Verification items for the finished model (mm, model axes). Face numbers are marked on the shaded views. Give positions to 0.01 mm unless a question says otherwise; leave off trailing zeros. Order: outer loops, then holes, each group sorted by start corner. A loop starts at its lowest first (then second) coordinate and runs counter-clockwise, first axis right, second up. Notation, with made-up numbers: (17.5, -37) -> (41.5, -37) arc R25 cw to (41.5, -16) -> close; hole circle Ø6 at (65, -8). An arc over 180 degrees is marked (long way). One line per question, with ' | ' between items. Start each with the question number.
Q1. Section check D-D on y = 12.75. Record the cut outline in (x, z), plus the area to 3 significant figures.
Q2. Section check C-C on z = 0. Record the cut outline in (x, y), plus the area to 3 significant figures.
Q3. Section check B-B on z = -20. Record the cut outline in (x, y), plus the area to 3 significant figures.
Q4. Material ranges on probe 1 along Z at (x, y) = (-2, 20.5); probe 2 along Y at (x, z) = (3.25, 0); probe 3 along Y at (x, z) = (4.75, -4), recorded low to high. Write a range as [from, to].
Q5. Go/stop test with flat-tipped pins: pin 1 (1 mm diameter, centred on x = 1.5, y = 17.5, fed in from +Z); pin 2 (1.3 mm diameter, centred on y = 20, z = -31, fed in from -X); pin 3 (8 mm diameter, centred on y = 6, z = -43, fed in from -X). Record where each tip stops, or that it passes through.
Q6. Section check A-A on z = 42. Record the cut outline in (x, y).
Q7. Mould release check, pull along X, two halves, no side actions. Record for the marked faces 1 and 2: released by +X, released by -X, zero draft, split by the parting line, or undercut.
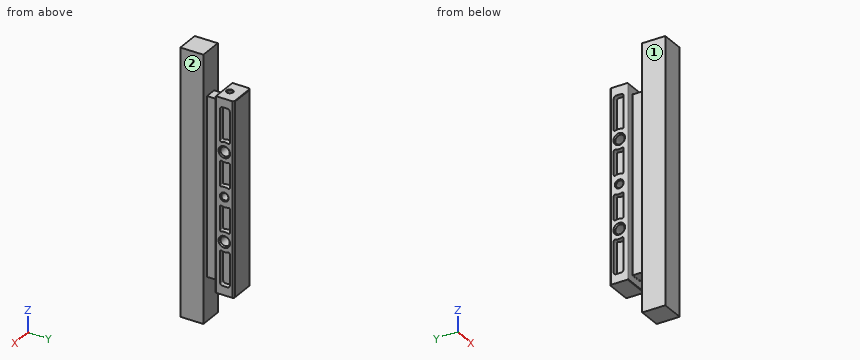
from build123d import *

# Parameters (mm, degrees)
BOSS_EXTRUDE1_DEPTH      = 60
BOSS_EXTRUDE1_DEPTH_BACK = 60
CUT_EXTRUDE1_DEPTH       = 12
CUT_EXTRUDE1_DEPTH_BACK  = 12
CUT_EXTRUDE2_DEPTH       = 2.3
CUT_EXTRUDE3_DEPTH       = 2.3
CUT_EXTRUDE4_DEPTH       = 2.3
CUT_EXTRUDE5_DEPTH       = 2.3
CUT_EXTRUDE6_DEPTH       = 2.3
CUT_EXTRUDE7_DEPTH       = 2.3
CUT_EXTRUDE8_DEPTH       = 2.3
CUT_EXTRUDE9_DEPTH       = 2.3


with BuildPart() as part:
    # Sketch1 → Boss-Extrude1 (new body, two sides)
    with BuildSketch(Plane.XY) as boss_extrude1_sk:
        with BuildLine():
            Line((-5.8, 16.5), (-2.9, 16.5))
            ThreePointArc((-2.9, 16.5), (-2.687867966, 16.412132034), (-2.6, 16.2))
            Line((-2.6, 16.2), (-2.6, 10.5))
            Line((-2.6, 10.5), (-5.25, 10.5))
            Line((-5.25, 10.5), (-5.25, 0))
            Line((-5.25, 0), (5.25, 0))
            Line((5.25, 0), (5.25, 10.5))
            Line((5.25, 10.5), (2.6, 10.5))
            Line((2.6, 10.5), (2.6, 16.2))
            ThreePointArc((2.6, 16.2), (2.687867966, 16.412132034), (2.9, 16.5))
            Line((2.9, 16.5), (5.8, 16.5))
            ThreePointArc((5.8, 16.5), (5.941421356, 16.558578644), (6, 16.7))
            Line((6, 16.7), (6, 24.3))
            Line((6, 24.3), (5.3, 25))
            Line((5.3, 25), (-5.3, 25))
            Line((-5.3, 25), (-6, 24.3))
            Line((-6, 24.3), (-6, 16.7))
            ThreePointArc((-6, 16.7), (-5.941421356, 16.558578644), (-5.8, 16.5))
        make_face()
    extrude(amount=BOSS_EXTRUDE1_DEPTH)
    extrude(boss_extrude1_sk.sketch, amount=-BOSS_EXTRUDE1_DEPTH_BACK)

    # Sketch2 → Cut-Extrude1 (cut, two sides)
    with BuildSketch(Plane(origin=(0, 0, 0), x_dir=(0, 0, -1), z_dir=(1, 0, 0))) as cut_extrude1_sk:
        with BuildLine():
            Line((-65, 30), (-65, 10.5))
            Line((-65, 10.5), (-40.3, 10.5))
            Line((-40.3, 10.5), (-40.3, 16.2))
            ThreePointArc((-40.3, 16.2), (-40.387867966, 16.412132034), (-40.6, 16.5))
            Line((-40.6, 16.5), (-43.6, 16.5))
            Line((-43.6, 16.5), (-43.8, 16.7))
            Line((-43.8, 16.7), (-43.8, 24.8))
            Line((-43.8, 24.8), (-43.6, 25))
            Line((-43.6, 25), (43.6, 25))
            Line((43.6, 25), (43.8, 24.8))
            Line((43.8, 24.8), (43.8, 16.7))
            Line((43.8, 16.7), (43.6, 16.5))
            Line((43.6, 16.5), (40.6, 16.5))
            ThreePointArc((40.6, 16.5), (40.387867966, 16.412132034), (40.3, 16.2))
            Line((40.3, 16.2), (40.3, 10.5))
            Line((40.3, 10.5), (65, 10.5))
            Line((65, 10.5), (65, 30))
            Line((65, 30), (-65, 30))
        make_face()
    extrude(amount=CUT_EXTRUDE1_DEPTH, mode=Mode.SUBTRACT)
    extrude(cut_extrude1_sk.sketch, amount=-CUT_EXTRUDE1_DEPTH_BACK, mode=Mode.SUBTRACT)

    # Sketch3 → Cut-Revolve1 (revolve, cut)
    with BuildSketch(Plane.XY):
        Polygon((-6, 20.5), (-6, 22.5), (-5.621, 22.121), (5.621, 22.121), (6, 22.5), (6, 20.5), align=None)
    revolve(axis=Axis((6, 20.5, 0), (-1, 0, 0)), mode=Mode.SUBTRACT)

    # Sketch4 → Cut-Revolve2 (revolve, cut)
    with BuildSketch(Plane.XY.offset(20)):
        Polygon((-6, 20.5), (-6, 23.15), (-5.454778834, 22.6), (5.454778834, 22.6), (6, 23.15), (6, 20.5), align=None)
    revolve(axis=Axis((0, 20.5, 20), (-1, 0, 0)), mode=Mode.SUBTRACT)

    # Sketch5 → Cut-Revolve3 (revolve, cut)
    with BuildSketch(Plane.XY.offset(-20)):
        Polygon((-6, 20.5), (-6, 23.15), (-5.454778834, 22.6), (5.454778834, 22.6), (6, 23.15), (6, 20.5), align=None)
    revolve(axis=Axis((0, 20.5, -20), (-1, 0, 0)), mode=Mode.SUBTRACT)

    # Sketch6 → Cut-Revolve4 (revolve, cut)
    with BuildSketch(Plane(origin=(0, 0, 0), x_dir=(0, 0, -1), z_dir=(1, 0, 0))):
        Polygon((-43.8, 19.3), (-43.8, 20.8), (-43.5295, 20.5295), (-33.3, 20.5295), (-32.590147844, 19.3), align=None)
    revolve(axis=Axis((0, 19.3, 32.590147844), (0, 0, 1)), mode=Mode.SUBTRACT)

    # Sketch7 → Cut-Extrude2 (cut)
    with BuildSketch(Plane(origin=(6, 0, 0), x_dir=(0, 0, -1), z_dir=(1, 0, 0))):
        with BuildLine():
            Line((24.698499761, 18.58), (38.8, 18.58))
            ThreePointArc((38.8, 18.58), (39.507106781, 18.872893219), (39.8, 19.58))
            Line((39.8, 19.58), (39.8, 22))
            ThreePointArc((39.8, 22), (39.507106781, 22.707106781), (38.8, 23))
            Line((38.8, 23), (24.698499761, 23))
            ThreePointArc((24.698499761, 23), (24.288926812, 22.786792608), (24.228649785, 22.329))
            ThreePointArc((24.228649785, 22.329), (24.5, 20.79), (24.228649785, 19.251))
            ThreePointArc((24.228649785, 19.251), (24.288926812, 18.793207392), (24.698499761, 18.58))
        make_face()
    extrude(amount=-CUT_EXTRUDE2_DEPTH, mode=Mode.SUBTRACT)

    # Sketch8 → Cut-Extrude3 (cut)
    with BuildSketch(Plane(origin=(6, 0, 0), x_dir=(0, 0, -1), z_dir=(1, 0, 0))):
        with BuildLine():
            Line((-39.8, 22), (-39.8, 19.58))
            ThreePointArc((-39.8, 19.58), (-39.507106781, 18.872893219), (-38.8, 18.58))
            Line((-38.8, 18.58), (-24.698499761, 18.58))
            ThreePointArc((-24.698499761, 18.58), (-24.288926812, 18.793207392), (-24.228649785, 19.251))
            ThreePointArc((-24.228649785, 19.251), (-24.5, 20.79), (-24.228649785, 22.329))
            ThreePointArc((-24.228649785, 22.329), (-24.288926812, 22.786792608), (-24.698499761, 23))
            Line((-24.698499761, 23), (-38.8, 23))
            ThreePointArc((-38.8, 23), (-39.507106781, 22.707106781), (-39.8, 22))
        make_face()
    extrude(amount=-CUT_EXTRUDE3_DEPTH, mode=Mode.SUBTRACT)

    # Sketch9 → Cut-Extrude4 (cut)
    with BuildSketch(Plane(origin=(6, 0, 0), x_dir=(0, 0, -1), z_dir=(1, 0, 0))):
        with BuildLine():
            Line((4.698499761, 18.58), (15.301500239, 18.58))
            ThreePointArc((15.301500239, 18.58), (15.711073188, 18.793207392), (15.771350215, 19.251))
            ThreePointArc((15.771350215, 19.251), (15.5, 20.79), (15.771350215, 22.329))
            ThreePointArc((15.771350215, 22.329), (15.711073188, 22.786792608), (15.301500239, 23))
            Line((15.301500239, 23), (4.698499761, 23))
            ThreePointArc((4.698499761, 23), (4.288926812, 22.786792608), (4.228649785, 22.329))
            ThreePointArc((4.228649785, 22.329), (4.5, 20.79), (4.228649785, 19.251))
            ThreePointArc((4.228649785, 19.251), (4.288926812, 18.793207392), (4.698499761, 18.58))
        make_face()
    extrude(amount=-CUT_EXTRUDE4_DEPTH, mode=Mode.SUBTRACT)

    # Sketch10 → Cut-Extrude5 (cut)
    with BuildSketch(Plane(origin=(6, 0, 0), x_dir=(0, 0, -1), z_dir=(1, 0, 0))):
        with BuildLine():
            Line((-15.301500239, 18.58), (-4.698499761, 18.58))
            ThreePointArc((-4.698499761, 18.58), (-4.288926812, 18.793207392), (-4.228649785, 19.251))
            ThreePointArc((-4.228649785, 19.251), (-4.5, 20.79), (-4.228649785, 22.329))
            ThreePointArc((-4.228649785, 22.329), (-4.288926812, 22.786792608), (-4.698499761, 23))
            Line((-4.698499761, 23), (-15.301500239, 23))
            ThreePointArc((-15.301500239, 23), (-15.711073188, 22.786792608), (-15.771350215, 22.329))
            ThreePointArc((-15.771350215, 22.329), (-15.5, 20.79), (-15.771350215, 19.251))
            ThreePointArc((-15.771350215, 19.251), (-15.711073188, 18.793207392), (-15.301500239, 18.58))
        make_face()
    extrude(amount=-CUT_EXTRUDE5_DEPTH, mode=Mode.SUBTRACT)

    # Sketch11 → Cut-Extrude6 (cut)
    with BuildSketch(Plane(origin=(-6, 0, 0), x_dir=(0, 0, -1), z_dir=(1, 0, 0))):
        with BuildLine():
            Line((24.698499761, 18.58), (38.8, 18.58))
            ThreePointArc((38.8, 18.58), (39.507106781, 18.872893219), (39.8, 19.58))
            Line((39.8, 19.58), (39.8, 22))
            ThreePointArc((39.8, 22), (39.507106781, 22.707106781), (38.8, 23))
            Line((38.8, 23), (24.698499761, 23))
            ThreePointArc((24.698499761, 23), (24.288926812, 22.786792608), (24.228649785, 22.329))
            ThreePointArc((24.228649785, 22.329), (24.5, 20.79), (24.228649785, 19.251))
            ThreePointArc((24.228649785, 19.251), (24.288926812, 18.793207392), (24.698499761, 18.58))
        make_face()
    extrude(amount=CUT_EXTRUDE6_DEPTH, mode=Mode.SUBTRACT)

    # Sketch12 → Cut-Extrude7 (cut)
    with BuildSketch(Plane(origin=(-6, 0, 0), x_dir=(0, 0, -1), z_dir=(1, 0, 0))):
        with BuildLine():
            Line((-39.8, 22), (-39.8, 19.58))
            ThreePointArc((-39.8, 19.58), (-39.507106781, 18.872893219), (-38.8, 18.58))
            Line((-38.8, 18.58), (-24.698499761, 18.58))
            ThreePointArc((-24.698499761, 18.58), (-24.288926812, 18.793207392), (-24.228649785, 19.251))
            ThreePointArc((-24.228649785, 19.251), (-24.5, 20.79), (-24.228649785, 22.329))
            ThreePointArc((-24.228649785, 22.329), (-24.288926812, 22.786792608), (-24.698499761, 23))
            Line((-24.698499761, 23), (-38.8, 23))
            ThreePointArc((-38.8, 23), (-39.507106781, 22.707106781), (-39.8, 22))
        make_face()
    extrude(amount=CUT_EXTRUDE7_DEPTH, mode=Mode.SUBTRACT)

    # Sketch13 → Cut-Extrude8 (cut)
    with BuildSketch(Plane(origin=(-6, 0, 0), x_dir=(0, 0, -1), z_dir=(1, 0, 0))):
        with BuildLine():
            Line((4.698499761, 18.58), (15.301500239, 18.58))
            ThreePointArc((15.301500239, 18.58), (15.711073188, 18.793207392), (15.771350215, 19.251))
            ThreePointArc((15.771350215, 19.251), (15.5, 20.79), (15.771350215, 22.329))
            ThreePointArc((15.771350215, 22.329), (15.711073188, 22.786792608), (15.301500239, 23))
            Line((15.301500239, 23), (4.698499761, 23))
            ThreePointArc((4.698499761, 23), (4.288926812, 22.786792608), (4.228649785, 22.329))
            ThreePointArc((4.228649785, 22.329), (4.5, 20.79), (4.228649785, 19.251))
            ThreePointArc((4.228649785, 19.251), (4.288926812, 18.793207392), (4.698499761, 18.58))
        make_face()
    extrude(amount=CUT_EXTRUDE8_DEPTH, mode=Mode.SUBTRACT)

    # Sketch14 → Cut-Extrude9 (cut)
    with BuildSketch(Plane(origin=(-6, 0, 0), x_dir=(0, 0, -1), z_dir=(1, 0, 0))):
        with BuildLine():
            Line((-15.301500239, 18.58), (-4.698499761, 18.58))
            ThreePointArc((-4.698499761, 18.58), (-4.288926812, 18.793207392), (-4.228649785, 19.251))
            ThreePointArc((-4.228649785, 19.251), (-4.5, 20.79), (-4.228649785, 22.329))
            ThreePointArc((-4.228649785, 22.329), (-4.288926812, 22.786792608), (-4.698499761, 23))
            Line((-4.698499761, 23), (-15.301500239, 23))
            ThreePointArc((-15.301500239, 23), (-15.711073188, 22.786792608), (-15.771350215, 22.329))
            ThreePointArc((-15.771350215, 22.329), (-15.5, 20.79), (-15.771350215, 19.251))
            ThreePointArc((-15.771350215, 19.251), (-15.711073188, 18.793207392), (-15.301500239, 18.58))
        make_face()
    extrude(amount=CUT_EXTRUDE9_DEPTH, mode=Mode.SUBTRACT)


solid = part.part
Filled in:
1) outline: (-2.6, -40.3) -> (2.6, -40.3) -> (2.6, 40.3) -> (-2.6, 40.3) -> close | area: 419 mm²
2) outline: (-6, 16.7) arc R0.2 ccw to (-5.8, 16.5) -> (-2.9, 16.5) arc R0.3 cw to (-2.6, 16.2) -> (-2.6, 10.5) -> (-5.25, 10.5) -> (-5.25, 0) -> (5.25, 0) -> (5.25, 10.5) -> (2.6, 10.5) -> (2.6, 16.2) arc R0.3 cw to (2.9, 16.5) -> (5.8, 16.5) arc R0.2 ccw to (6, 16.7) -> (6, 18.5) -> (5.62, 18.88) -> (-5.62, 18.88) -> (-6, 18.5) -> close; (-6, 22.5) -> (-5.62, 22.12) -> (5.62, 22.12) -> (6, 22.5) -> (6, 24.3) -> (5.3, 25) -> (-5.3, 25) -> (-6, 24.3) -> close | area: 204 mm²
3) outline: (-6, 16.7) arc R0.2 ccw to (-5.8, 16.5) -> (-2.9, 16.5) arc R0.3 cw to (-2.6, 16.2) -> (-2.6, 10.5) -> (-5.25, 10.5) -> (-5.25, 0) -> (5.25, 0) -> (5.25, 10.5) -> (2.6, 10.5) -> (2.6, 16.2) arc R0.3 cw to (2.9, 16.5) -> (5.8, 16.5) arc R0.2 ccw to (6, 16.7) -> (6, 17.85) -> (5.45, 18.4) -> (-5.45, 18.4) -> (-6, 17.85) -> close; (-6, 23.15) -> (-5.45, 22.6) -> (5.45, 22.6) -> (6, 23.15) -> (6, 24.3) -> (5.3, 25) -> (-5.3, 25) -> (-6, 24.3) -> close | area: 192 mm²
4) probe 1: [-43.8, -22.1], [-17.9, -1.62], [1.62, 17.9], [22.1, 43.8] | probe 2: [0, 10.5], [16.5, 18.88], [22.12, 25] | probe 3: [0, 10.5], [16.5, 25]
5) pin 1: z = 43.8 | pin 2: x = -3.7 | pin 3: x = -5.25
6) outline: (-6, 16.7) arc R0.2 ccw to (-5.8, 16.5) -> (5.8, 16.5) arc R0.2 ccw to (6, 16.7) -> (6, 24.3) -> (5.3, 25) -> (-5.3, 25) -> (-6, 24.3) -> close; (-5.25, 0) -> (5.25, 0) -> (5.25, 10.5) -> (-5.25, 10.5) -> close; hole circle Ø2.46 at (0, 19.3)
7) face 1: released by -X | face 2: released by +X
